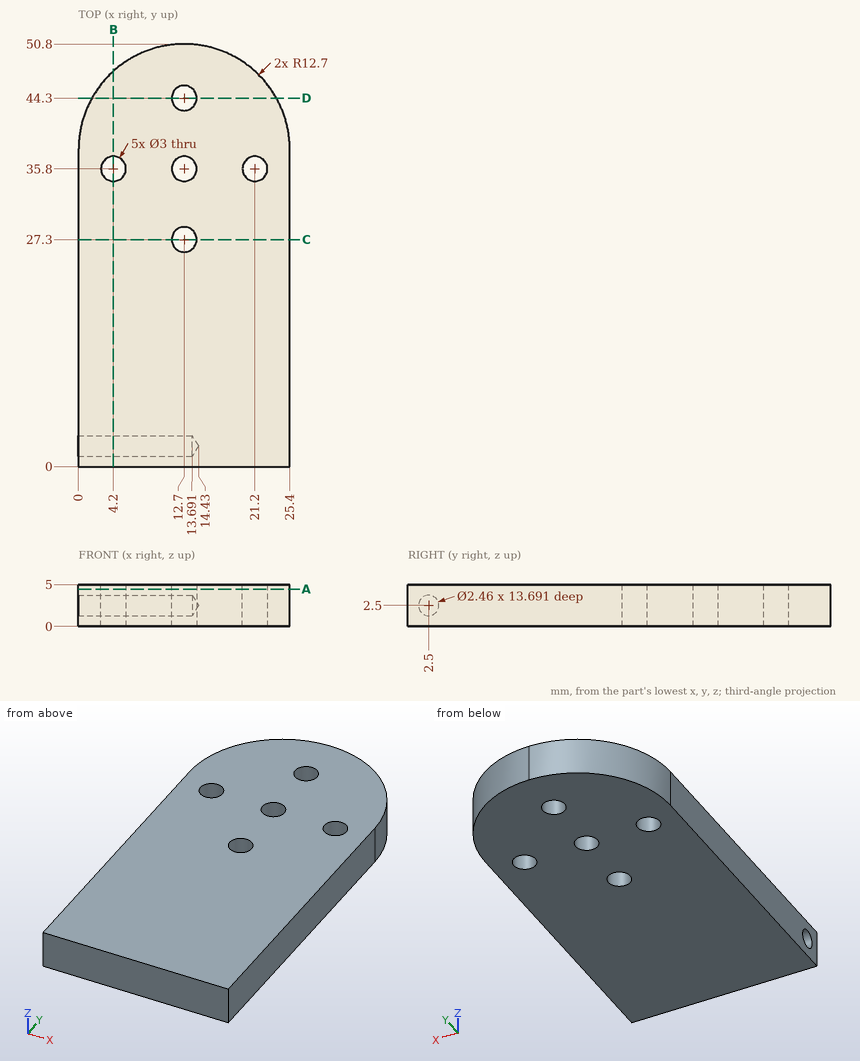
The drawing under review shows one solid part. Ordinate dimensions are in mm from its lowest x, y, z. Round coordinates to 2 decimals unless told otherwise and drop trailing zeros. Order: outer loops, then holes, each group sorted by start corner. A loop starts at its lowest first (then second) coordinate and runs counter-clockwise, first axis right, second up. Notation, with made-up numbers: (-7.75, -24.5) -> (-0.75, -24.5) arc R16 cw to (-0.75, -5.5) -> close; hole circle Ø10 at (61, 20). An arc over 180 degrees is marked (long way). Use a Markdown table: item, result.
Q1. We need section C-C on y = 27.3. Write out the cut boundary in (x, z).
Values:
| item | result |
|---|---|
| outline | (0, 0) -> (11.2, 0) -> (11.2, 5) -> (0, 5) -> close; (14.2, 0) -> (25.4, 0) -> (25.4, 5) -> (14.2, 5) -> close |
Q2. We need section D-D on y = 44.3. Write out the cut boundary in (x, z).
Values:
| item | result |
|---|---|
| outline | (1.62, 0) -> (11.2, 0) -> (11.2, 5) -> (1.62, 5) -> close; (14.2, 0) -> (23.78, 0) -> (23.78, 5) -> (14.2, 5) -> close |
Q3. For line 1 (Y direction, x = 12.7, z = 1.15); line 2 (X direction, y = 35, z = 2.15); line 3 (Y direction, x = 12, z = 2.55) (1 decimal), list the stretches that pass through material, from the lowest coordinate up.
Values:
| item | result |
|---|---|
| line 1 | y = 0 to 25.8, 28.8 to 34.3, 37.3 to 42.8, 45.8 to 50.8 |
| line 2 | x = 0 to 2.93, 5.47 to 11.43, 13.97 to 19.93, 22.47 to 25.4 |
| line 3 | y = 0 to 1.3, 3.7 to 26, 28.6 to 34.5, 37.1 to 43, 45.6 to 50.8 |
Q4. We need section B-B on x = 4.2. Write out the cut boundary in (y, z).
Values:
| item | result |
|---|---|
| outline | (0, 0) -> (34.3, 0) -> (34.3, 5) -> (0, 5) -> close; (37.3, 0) -> (47.54, 0) -> (47.54, 5) -> (37.3, 5) -> close; hole circle Ø2.46 at (2.5, 2.5) |
Q5. We need section A-A on z = 4.45. State how many separate pieces and enclosed holes the cut face has, then the cut area to 3 significant figures.
Values:
| item | result |
|---|---|
| separate pieces | 1 |
| enclosed holes | 5 |
| area | 1,190 mm^2 |
Q6. Clearance check with flat-ended pins moving along their axes: P1, Ø1, axis at x = 11.5, z = 3, coming from the +Y side; P2, Ø5, axis at x = 21.2, y = 35.8, coming from the -Z side. State where each tip first meets the part, or that it passes through.
Values:
| item | result |
|---|---|
| P1 | stops at y = 50.78 |
| P2 | stops at z = 0 |
